Source: CAD feature listing. Evaluate the final solid. Frame: model axes, mm. Face numbers are marked on the shaded views. A direction names the side the tool comes from. Give positions to 0.01 mm unless a question says otherwise; leave off trailing zeros. Order: outer loops, then holes, each group sorted by start corner. A loop starts at its lowest first (then second) coordinate and runs counter-clockwise, first axis right, second up. Notation, with made-up numbers: M 46.25,74 L 98.25,74 A16 ccw 98.25,87 Z; hole C -18,30.5 d3. An arc over 180 degrees is marked long. Answer as a JSON object with one key per item and string values. Group by question number.
1. Pin query (flat end, axial travel): P1, Ø12, axis at x = 191, y = 78, coming from the +Z side (3 decimals); P2, Ø4, axis at y = 170.5, z = 74, coming from the +X side; P3, Ø10, axis at x = 1, z = 76.5, coming from the +Y side. Return the tip coordinate at first contact, or that it passes through.
2. Set-up query: the marked faces 1, 2, 3 and 4. Return all of +Z, -Z, +X, -X, +Y, -Y with unobstructed straight access to the full face (end or side cutting, diameter ignored); none if empty.
3. Material intervals for L1, parallel to Y at x = 152.5, z = -29; L2, parallel to Y at x = 38, z = 70; L3, parallel to Z at x = -17, y = 149, sorted ascending. Write a range as [from, to].
4. Section query D-D (z = 83.5). Output: boundary loops of the cut face in (x, y).
5. Section query B-B (y = 142). Output: boundary loops of the cut face in (x, z).
6. Section query C-C (x = 32.5). Output: boundary loops of the cut face in (y, z).
7. Section query A-A (z = 37.5). Output: boundary loops of the cut face in (x, y).
from build123d import *

# Parameters (mm, degrees)
SKETCH1_W      = 309.88
SKETCH1_H      = 136.398
EXTRUDE1_DEPTH = 160.528
SKETCH2_R      = 54.23826071
EXTRUDE2_DEPTH = 81.534
SKETCH3_R      = 76.2
EXTRUDE3_DEPTH = 19.812


with BuildPart() as part:
    # Sketch1 → Extrude1 (new body)
    with BuildSketch(Plane(origin=(0, 0, 0), x_dir=(1, 0, 0), z_dir=(0, 1, 0))):
        with Locations((120.827186097, -35.645984436)):
            Rectangle(SKETCH1_W, SKETCH1_H)
    extrude(amount=EXTRUDE1_DEPTH)

    # Sketch2 → Extrude2 (add)
    with BuildSketch(Plane(origin=(0, 160.528, 0), x_dir=(1, 0, 0), z_dir=(0, 1, 0))):
        with Locations(Location((126.415186097, -35.645984436, 0), (0, 0, 270))):
            Circle(SKETCH2_R)
    extrude(amount=EXTRUDE2_DEPTH)

    # Sketch3 → Extrude3 (add)
    with BuildSketch(Plane(origin=(0, 242.062, 0), x_dir=(1, 0, 0), z_dir=(0, 1, 0))):
        with Locations(Location((126.415186097, -35.645984436, 0), (0, 0, 270))):
            Circle(SKETCH3_R)
    extrude(amount=-EXTRUDE3_DEPTH)


solid = part.part
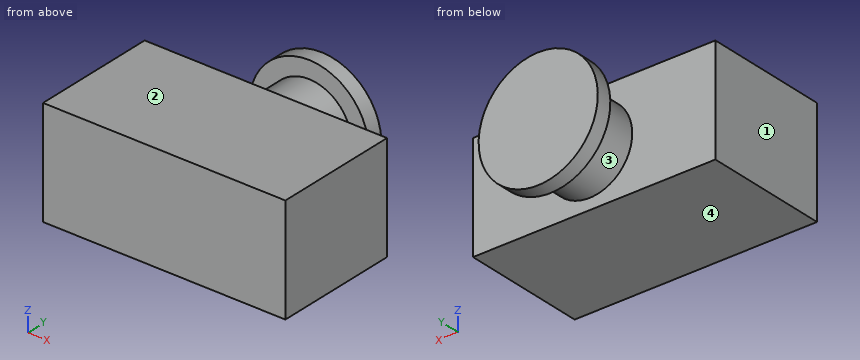
Answer sheet:
{
 "1": {"P1": "z = 103.845", "P2": "x = 166.67", "P3": "y = 160.53"},
 "2": {"face 1": "+Z, -Z, -X, +Y, -Y", "face 2": "+Z, +X, -X, -Y", "face 3": "none", "face 4": "-Z, +X, -X, -Y"},
 "3": {"L1": "[0, 160.53], [222.25, 242.06]", "L2": "[0, 160.53]", "L3": "[-32.55, 103.84]"},
 "4": {"outline": "M -34.11,0 L 275.77,0 L 275.77,160.53 L 151.95,160.53 L 151.95,222.25 L 185.71,222.25 L 185.71,242.06 L 67.12,242.06 L 67.12,222.25 L 100.89,222.25 L 100.89,160.53 L -34.11,160.53 Z"},
 "5": {"outline": "M -34.11,-32.55 L 275.77,-32.55 L 275.77,103.84 L -34.11,103.84 Z"},
 "6": {"outline": "M 0,-32.55 L 160.53,-32.55 L 160.53,103.84 L 0,103.84 Z"},
 "7": {"outline": "M -34.11,0 L 275.77,0 L 275.77,160.53 L 180.62,160.53 L 180.62,222.25 L 202.59,222.25 L 202.59,242.06 L 50.24,242.06 L 50.24,222.25 L 72.21,222.25 L 72.21,160.53 L -34.11,160.53 Z"}
}
